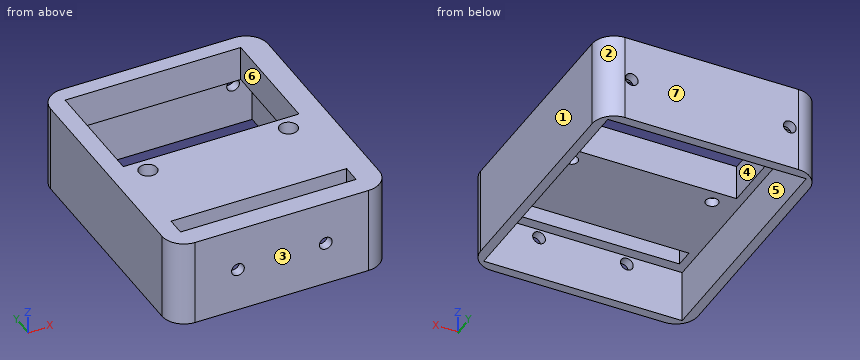
from build123d import *

# Parameters (mm, degrees)
EXTRUDE_1_DEPTH     = 20
SKETCH_2_W          = 45.2
SKETCH_2_H          = 55.2
CUT_EXTRUDE_1_DEPTH = 12
SKETCH_4_W          = 40
SKETCH_4_H          = 25.9
SKETCH_4_H_2        = 4.2
CUT_EXTRUDE_2_DEPTH = 21
SKETCH_6_R          = 1.45
CUT_EXTRUDE_4_DEPTH = 9
SKETCH_7_R          = 2.05
CUT_EXTRUDE_5_DEPTH = 6
SKETCH_8_R          = 1.45
CUT_EXTRUDE_6_DEPTH = 6
SKETCH_9_R          = 1.45
CUT_EXTRUDE_7_DEPTH = 6


with BuildPart() as part:
    # 草图1 → 凸台-拉伸1 (new body)
    with BuildSketch(Plane.XY):
        with BuildLine():
            Line((-19.75, 29.75), (19.75, 29.75))
            ThreePointArc((19.75, 29.75), (23.285533906, 28.285533906), (24.75, 24.75))
            Line((24.75, 24.75), (24.75, -24.75))
            ThreePointArc((24.75, -24.75), (23.285533906, -28.285533906), (19.75, -29.75))
            Line((19.75, -29.75), (-19.75, -29.75))
            ThreePointArc((-19.75, -29.75), (-23.285533906, -28.285533906), (-24.75, -24.75))
            Line((-24.75, -24.75), (-24.75, 24.75))
            ThreePointArc((-24.75, 24.75), (-23.285533906, 28.285533906), (-19.75, 29.75))
        make_face()
    extrude(amount=EXTRUDE_1_DEPTH)

    # 草图2 → 切除-拉伸1 (cut)
    with BuildSketch(Plane(origin=(0, 0, 0), x_dir=(-1, 0, 0), z_dir=(0, 0, -1))):
        Rectangle(SKETCH_2_W, SKETCH_2_H)
    extrude(amount=-CUT_EXTRUDE_1_DEPTH, mode=Mode.SUBTRACT)

    # 草图4 → 切除-拉伸2 (cut, through all)
    with BuildSketch(Plane.XY.offset(20)):
        with Locations((-0.75, 13.2)):
            Rectangle(SKETCH_4_W, SKETCH_4_H)
        with Locations((-0.75, -23.065049662)):
            Rectangle(SKETCH_4_W, SKETCH_4_H_2)
    extrude(amount=-CUT_EXTRUDE_2_DEPTH, mode=Mode.SUBTRACT)

    # 草图6 → 切除-拉伸4 (cut, through all)
    with BuildSketch(Plane(origin=(0, 0, 12), x_dir=(-1, 0, 0), z_dir=(0, 0, -1))):
        with Locations((16.862, -3.116)):
            Circle(SKETCH_6_R)
        with Locations((-15.138, -3.116)):
            Circle(SKETCH_6_R)
    extrude(amount=-CUT_EXTRUDE_4_DEPTH, mode=Mode.SUBTRACT)

    # 草图7 → 切除-拉伸5 (cut)
    with BuildSketch(Plane.XY.offset(20)):
        with Locations((-16.862, -3.116)):
            Circle(SKETCH_7_R)
        with Locations((15.138, -3.116)):
            Circle(SKETCH_7_R)
    extrude(amount=-CUT_EXTRUDE_5_DEPTH, mode=Mode.SUBTRACT)

    # 草图8 → 切除-拉伸6 (cut)
    with BuildSketch(Plane(origin=(0, 29.75, 0), x_dir=(1, 0, 0), z_dir=(0, 1, 0))):
        with Locations((-17.75, -10)):
            Circle(SKETCH_8_R)
        with Locations((18.25, -10)):
            Circle(SKETCH_8_R)
    extrude(amount=-CUT_EXTRUDE_6_DEPTH, mode=Mode.SUBTRACT)

    # 草图9 → 切除-拉伸7 (cut)
    with BuildSketch(Plane.XZ.offset(29.75)):
        with Locations((-10, 10)):
            Circle(SKETCH_9_R)
        with Locations((10, 10)):
            Circle(SKETCH_9_R)
    extrude(amount=-CUT_EXTRUDE_7_DEPTH, mode=Mode.SUBTRACT)


solid = part.part
Can you work these out from the model? Positions are in its coordinate system, mm. Face numbers are marked on the shaded views. A direction names the side the tool comes from. Round coordinates to 2 decimals unless told otherwise and drop trailing zeros. Write each loop counter-clockwise with the first axis right and the second up, starting at its lowest first coordinate (ties: lowest second). Pieces come first, ordered by that corner, then holes. Notation, with made-up numbers: M 36.25,31.5 L 63.25,31.5 A14 ccw 63.25,41.5 Z; hole C 83,21.25 d1. An arc over 180 degrees is marked long. Use CSV: the item, a comma, the result in double quotes.
(1) Imagine slicing it at D-D (z = 4.5). Write out the boundary of the cut face in (x, y).
Check values:
outline,"M -24.75,-24.75 A5 ccw -19.75,-29.75 L 19.75,-29.75 A5 ccw 24.75,-24.75 L 24.75,24.75 A5 ccw 19.75,29.75 L -19.75,29.75 A5 ccw -24.75,24.75 Z; hole M -22.6,-27.6 L 22.6,-27.6 L 22.6,27.6 L -22.6,27.6 Z"
(2) I'm going to push flat-ended pins straight in: pin 1 (2 mm diameter, centred on x = 10, y = -9, fed in from -Z); pin 2 (4 mm diameter, centred on x = 15.138, y = -3.116, fed in from +Z); pin 3 (2 mm diameter, centred on x = -18, y = -2, fed in from +Z); pin 4 (2.5 mm diameter, centred on x = 18.25, z = 10, fed in from +Y). Where does each tip first touch, or does it pass through?
Check values:
pin 1,"z = 12"
pin 2,"z = 14"
pin 3,"z = 20"
pin 4,"y = -27.6"
(3) I need wall thicknesses on line 1 along Y through (x, z) = (-10, 13.25); line 2 along X through (y, z) = (-20, 2); line 3 along Y through (x, z) = (14, 4.25). Which ranges of each line are inside material? Lowest first, please.
Check values:
line 1,"-29.75 to -25.17, -20.97 to 0.25, 26.15 to 29.75"
line 2,"-24.75 to -22.6, 22.6 to 24.75"
line 3,"-29.75 to -27.6, 27.6 to 29.75"
(4) We'd pull the mould along Y, two halves only. Please class the marked faces 1, 2, 3 and 4: +Y half, -Y half, draft (parallel to the pull), parting line (faces both ways), or undercut.
Check values:
face 1,"draft"
face 2,"+Y half"
face 3,"-Y half"
face 4,"undercut"
(5) Imagine slicing it at A-A (x = -3.5). Write out the boundary of the cut face in (y, z).
Check values:
outline,"M -29.75,0 L -27.6,0 L -27.6,12 L -25.17,12 L -25.17,20 L -29.75,20 Z; M -20.97,12 L 0.25,12 L 0.25,20 L -20.97,20 Z; M 26.15,12 L 27.6,12 L 27.6,0 L 29.75,0 L 29.75,20 L 26.15,20 Z"
(6) Imagine slicing it at C-C (y = 15). Write out the boundary of the cut face in (x, z), plus the area to 3 significant figures.
Check values:
outline,"M -24.75,0 L -22.6,0 L -22.6,12 L -20.75,12 L -20.75,20 L -24.75,20 Z; M 19.25,12 L 22.6,12 L 22.6,0 L 24.75,0 L 24.75,20 L 19.25,20 Z"
area,"128 mm^2"
(7) Imagine slicing it at B-B (z = 10). Write out the boundary of the cut face in (x, y).
Check values:
outline,"M -24.75,-24.75 A5 ccw -19.75,-29.75 L -11.45,-29.75 L -11.45,-27.6 L -22.6,-27.6 L -22.6,27.6 L -19.2,27.6 L -19.2,29.75 L -19.75,29.75 A5 ccw -24.75,24.75 Z; M -16.3,27.6 L 16.8,27.6 L 16.8,29.75 L -16.3,29.75 Z; M -8.55,-29.75 L 8.55,-29.75 L 8.55,-27.6 L -8.55,-27.6 Z; M 11.45,-29.75 L 19.75,-29.75 A5 ccw 24.75,-24.75 L 24.75,24.75 A5 ccw 19.75,29.75 L 19.7,29.75 L 19.7,27.6 L 22.6,27.6 L 22.6,-27.6 L 11.45,-27.6 Z"
(8) On a 3-axis mill with a long thin cutter (end or side, diameter ignored), from which of +Z, -Z, +X, -X, +Y, -Y can I reach the whole of each face in a straight line? I mean the marked faces 5, 6 and 7. Say none if no direction works.
Check values:
face 5,"-Z"
face 6,"+Z, -Z"
face 7,"+Z, -Z, +X, -X, +Y"
